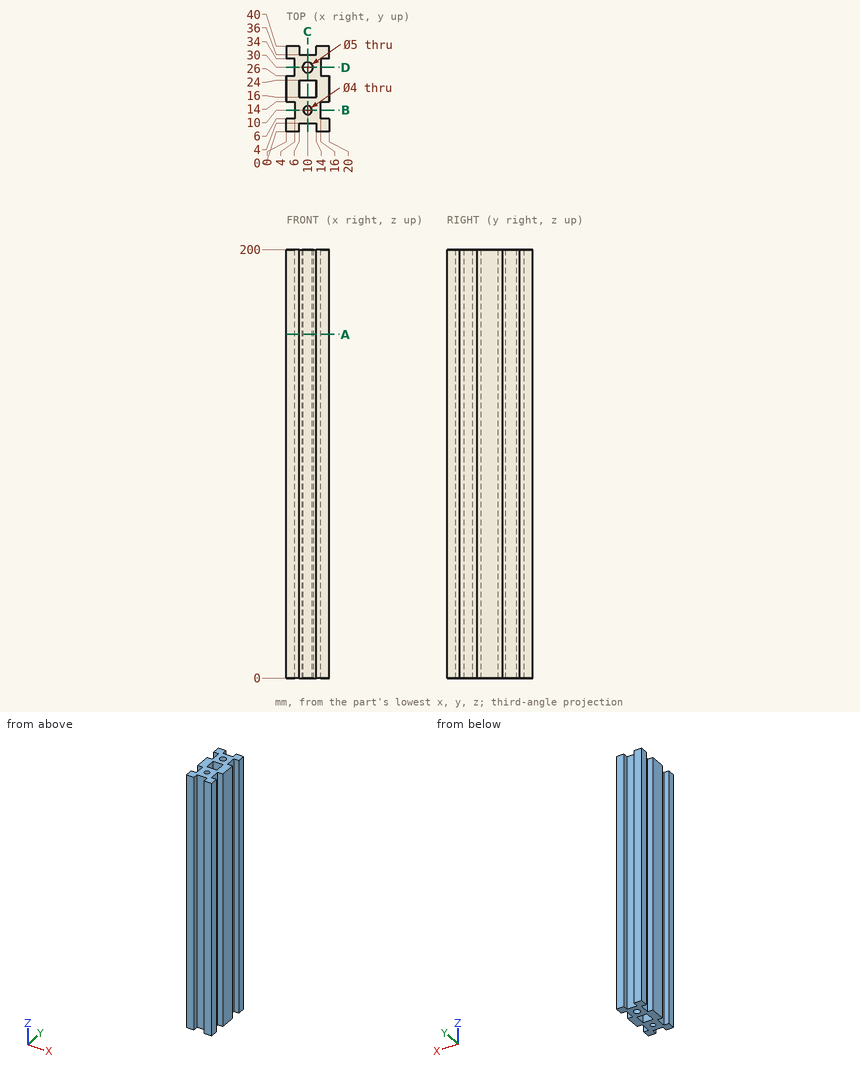
Source: three-view drawing plus pictorial views. Frame: mm from the lowest corner of the part. Coordinates: 2 decimals unless noted, no trailing zeros. Order: outer loops, then holes, each group sorted by start corner. A loop starts at its lowest first (then second) coordinate and runs counter-clockwise, first axis right, second up. Notation, with made-up numbers: M 12,-26.75 L 44,-26.75 A23 ccw 44,-12.75 Z; hole C 22.5,85.25 d10. An arc over 180 degrees is marked long. Write each question's results on one line, items separated by ' | '. Start each with the question number.
1. Section A-A, the plane z = 160.5. State how many separate pieces and enclosed holes the cut face has, then the cut area to 3 significant figures.
2. Pin query (flat end, axial travel): pin 1 (6.5 mm diameter, centred on x = 10, z = 59.5, fed in from +Y); pin 2 (1.5 mm diameter, centred on x = 2.5, y = 12.5, fed in from +Z); pin 3 (1 mm diameter, centred on y = 32, z = 69, fed in from +X). Return the tip coordinate at first contact, or that it passes through.
3. Material intervals for L1, parallel to Y at x = 10, z = 133; L2, parallel to Y at x = 2.5, z = 152.5; L3, parallel to Y at x = 9.5, z = 67, sorted ascending.
4. Section B-B, the plane y = 10. Return the cut outline in (x, z).
5. Section C-C, the plane x = 10. Return the cut outline in (y, z), then the cut area to 3 significant figures.
6. Section D-D, the plane y = 30. Return the cut outline in (x, z), then the cut area to 3 significant figures.
Solution:
1) separate pieces: 1 | enclosed holes: 3 | area: 512 mm²
2) pin 1: y = 36 | pin 2: through | pin 3: x = 16
3) L1: 4 to 8, 12 to 16, 24 to 27.5, 32.5 to 36 | L2: 0 to 6, 14 to 26, 34 to 40 | L3: 4 to 8.06, 11.94 to 16, 24 to 27.55, 32.45 to 36
4) outline: M 4,0 L 8,0 L 8,200 L 4,200 Z; M 12,0 L 16,0 L 16,200 L 12,200 Z
5) outline: M 4,0 L 8,0 L 8,200 L 4,200 Z; M 12,0 L 16,0 L 16,200 L 12,200 Z; M 24,0 L 27.5,0 L 27.5,200 L 24,200 Z; M 32.5,0 L 36,0 L 36,200 L 32.5,200 Z | area: 3,000 mm²
6) outline: M 4,0 L 7.5,0 L 7.5,200 L 4,200 Z; M 12.5,0 L 16,0 L 16,200 L 12.5,200 Z | area: 1,400 mm²
